The model under review builds one solid part; all positions refer to its coordinate system, in mm. A direction names the side the tool comes from. Give positions to 0.01 mm unless a question says otherwise; leave off trailing zeros. Loops run counter-clockwise (first coordinate to the right, second up) from the corner with the lowest first, then second, coordinate; pieces in that order, holes last. Notation, with made-up numbers: (77.5, 5) - (123.5, 5) arc R21 cw to (123.5, 44) - close; hole circle Ø11 at (25, -3). An arc over 180 degrees is marked (long way). Return JSON: item names as keys, results as strings. Group by question number.
from build123d import *

# Parameters (mm, degrees)
F1_DEPTH = 4


with BuildPart() as f1:
    # F0 (on Front) → F1 (new body)
    with BuildSketch(Plane.XZ):
        Polygon((0, 11.8332719468), (-8.6397333108, 11.8332719468), (-8.6397333108, 6.7300641264), (-8.6397333108, 0.1404409475), (-8.6397333108, -5.1667280532), (-0.1397333108, -5.1667280532), align=None)
        Polygon((8.3602666892, 11.8332719468), (0, 11.8332719468), (-0.1397333108, -5.1667280532), (8.3602666892, -5.1667280532), (8.3602666892, 0), (8.3602666892, 6.5887328237), align=None)
        with BuildLine():
            Line((-8.6397333108, 0.1404409475), (-8.6397333108, 6.7300641264))
            Line((-8.6397333108, 6.7300641264), (-15.9138074311, 6.8496522601))
            ThreePointArc((-15.9138074311, 6.8496522601), (-14.0683365047, 5.6735222105), (-13.3499665501, 3.6064011588))
            ThreePointArc((-13.3499665501, 3.6064011588), (-14.2983442905, 1.2776715705), (-16.6038153702, 0.2740755688))
            Line((-16.6038153702, 0.2740755688), (-16.6038047398, 0.2713728604))
            Line((-16.6038047398, 0.2713728604), (-8.6397333108, 0.1404409475))
        make_face()
        with BuildLine():
            ThreePointArc((-13.3499665501, 3.6064011588), (-14.0683365047, 5.6735222105), (-15.9138074311, 6.8496522601))
            Line((-15.9138074311, 6.8496522601), (-16.6297248975, 6.8614221751))
            Line((-16.6297248975, 6.8614221751), (-16.6038153702, 0.2740755688))
            ThreePointArc((-16.6038153702, 0.2740755688), (-14.2983442905, 1.2776715705), (-13.3499665501, 3.6064011588))
        make_face()
        with BuildLine():
            Line((-16.6297248975, 6.8614221751), (-15.9138074311, 6.8496522601))
            ThreePointArc((-15.9138074311, 6.8496522601), (-19.9983087172, 3.954267951), (-16.6038153702, 0.2740755688))
            Line((-16.6038153702, 0.2740755688), (-16.6297248975, 6.8614221751))
        make_face()
        with BuildLine():
            Line((15.8297359903, 6.5887328237), (8.3602666892, 6.5887328237))
            Line((8.3602666892, 6.5887328237), (8.3602666892, 0))
            Line((8.3602666892, 0), (16.4115056396, 0))
            Line((16.4115056396, 0), (16.4115606959, 0.0027021685))
            ThreePointArc((16.4115606959, 0.0027021685), (13.2254096253, 3.0399456203), (15.8297359903, 6.5887328237))
        make_face()
        with BuildLine():
            Line((16.5457502007, 6.5887328237), (15.8297359903, 6.5887328237))
            ThreePointArc((15.8297359903, 6.5887328237), (13.2254096253, 3.0399456203), (16.4115606959, 0.0027021685))
            Line((16.4115606959, 0.0027021685), (16.5457502007, 6.5887328237))
        make_face()
        with BuildLine():
            ThreePointArc((19.8790221475, 3.3332719468), (18.634294166, 5.9310952618), (15.8297359903, 6.5887328237))
            Line((15.8297359903, 6.5887328237), (16.5457502007, 6.5887328237))
            Line((16.5457502007, 6.5887328237), (16.4115606959, 0.0027021685))
            ThreePointArc((16.4115606959, 0.0027021685), (18.8547988965, 0.929317706), (19.8790221475, 3.3332719468))
        make_face()
    extrude(amount=F1_DEPTH)


solid = f1.part
Item 1: Take a section at C-C (z = 9.25). State the section outline as (x, y) points, then the cut area to 3 significant figures.
Item 2: Mouldability with a two-part tool opening along X and no side actions: class faces 1 (the face through (-8.64, -2, -2)), 2 (the face through (8.36, -2, -3)), 3 (the face through (0, 0, 3)), 4 (the face through (12, -2, 6.589)) as +X half, -X half, draft (parallel to the pull), parting line (faces both ways), or undercut.
Item 3: Tool access review of faces 5 (the face through (12, -2, 0)), 6 (the face through (0, -2, -5.167)): name each direction out of +Z, -Z, +X, -X, +Y, -Y from which nothing blocks a thin tool from reaching the whole face with its end or side.
Item 4: Take a section at B-B (x = 14.5). State the section outline as (y, z) points.
Item 5: For L1, parallel to Z at x = 9, y = -1.4; L2, parallel to X at y = -1.9, z = 11; L3, parallel to Z at x = -16.5, y = -2.6, list the stretches that pass through material, from the lowest coordinate up. Write a range as from..to.
Item 6: For P1, Ø1.5, axis at y = -3.5, z = 7, coming from the +X side; P2, Ø2, axis at y = -2.5, z = -3, coming from the -X side; P3, Ø1.2, axis at x = 13.5, y = -2, coming from the -Z side, all flat-tipped, find the tip position at first contact; note any pin that passes through.
Check sheet entries:
{
 "1": {"outline": "(-8.64, -4) - (8.36, -4) - (8.36, 0) - (-8.64, 0) - close", "area": "68.0 mm^2"},
 "2": {"face 1": "-X half", "face 2": "+X half", "face 3": "draft", "face 4": "undercut"},
 "3": {"face 5": "-Z, +X, +Y, -Y", "face 6": "-Z, +X, -X, +Y, -Y"},
 "4": {"outline": "(-4, 0) - (0, 0) - (0, 6.59) - (-4, 6.59) - close"},
 "5": {"L1": "z = 0..6.59", "L2": "x = -8.64..8.36", "L3": "z = 0.27..6.93"},
 "6": {"P1": "stops at x = 18.16", "P2": "stops at x = -8.64", "P3": "stops at z = 0"}
}
